```python
from build123d import *

# Parameters (mm, degrees)
F0_W     = 25.4
F0_H     = 25.4
F1_DEPTH = 44.45
F2_R     = 4.7625
F3_DEPTH = 25.401
F4_R     = 1.5875
F5_DEPTH = 12.7
F6_R     = 3.175
F7_DEPTH = 12.7


with BuildPart() as f1:
    # F0 (on Top) → F1 (new body)
    with BuildSketch(Plane.XY):
        Rectangle(F0_W, F0_H)
    extrude(amount=F1_DEPTH)

    # F2 (on face) → F3 (cut, through all)
    with BuildSketch(Plane.XZ.offset(12.7)):
        with Locations((0, 22.225)):
            Circle(F2_R)
    extrude(amount=-F3_DEPTH, mode=Mode.SUBTRACT)

    # F4 (on face) → F5 (cut)
    with BuildSketch(Plane.YZ.offset(12.7)):
        with Locations((0, 22.225)):
            Circle(F4_R)
    extrude(amount=-F5_DEPTH, mode=Mode.SUBTRACT)

    # F6 (on face) → F7 (cut)
    with BuildSketch(Plane(origin=(-12.7, 0, 0), x_dir=(0, -1, 0), z_dir=(-1, 0, 0))):
        with Locations((0, 33.3375)):
            Circle(F6_R)
        with Locations((0, 11.1125)):
            Circle(F6_R)
    extrude(amount=-F7_DEPTH, mode=Mode.SUBTRACT)


solid = f1.part
```
Geometry: final body of the model. Coordinates: model frame, mm. A direction names the side the tool comes from. Coordinates: 2 decimals unless noted, no trailing zeros. Order: outer loops, then holes, each group sorted by start corner. A loop starts at its lowest first (then second) coordinate and runs counter-clockwise, first axis right, second up. Notation, with made-up numbers: (-12, 22) - (37, 22) arc R13 ccw to (37, 47) - close; hole circle Ø5 at (4.25, 75.25). An arc over 180 degrees is marked (long way). Write each question's results on one line, items separated by ' | '.
1) Line query: line 1 (Z direction, x = 0, y = 5.75); line 2 (Z direction, x = 10.25, y = 0); line 3 (X direction, y = 6.5, z = 18). Output: solid intervals per line, ascending. Write a range as from..to.
Results list:
line 1: 0..17.46, 26.99..44.45 | line 2: 0..20.64, 23.81..44.45 | line 3: -12.7..-2.2, 2.2..12.7
2) Section B-B, the plane x = -3.25. State how many separate pieces and enclosed holes the cut face has, plus the area to 3 significant figures.
Results list:
separate pieces: 2 | enclosed holes: 2 | area: 889 mm^2
3) Section A-A, the plane x = 3.25. Return loops of the section in (y, z).
Results list:
outline: (-12.7, 0) - (12.7, 0) - (12.7, 18.74) - (-12.7, 18.74) - close; (-12.7, 25.71) - (12.7, 25.71) - (12.7, 44.45) - (-12.7, 44.45) - close
4) Pin query (flat end, axial travel): pin 1 (1.9 mm diameter, centred on y = 1, z = 10.5, fed in from -X). Return the tip coordinate at first contact, or that it passes through.
Results list:
pin 1: x = 0
5) Pull-direction query (Z, two-part tool) for faces 4 (the flat face through (0, 0, 44.45)), 5 (the flat face through (0, 0, 11)), 6 (the flat face through (-12.7, 0, 22)); classes: pulls with the +Z half, pulls with the -Z half, needs draft (parallel to the pull), parting line crosses it, or undercut.
Results list:
face 4: pulls with the +Z half | face 5: undercut | face 6: needs draft
6) Set-up query: faces 1 (the cylindrical face through (-6.439, 0.688, 8.013)), 2 (the cylindrical face through (8.652, 0.853, 23.564)), 3 (the cylindrical face through (-4.76, -0.18, 22.43)). Return all of +Z, -Z, +X, -X, +Y, -Y with unobstructed straight access to the full face (end or side cutting, diameter ignored); none if empty.
Results list:
face 1: -X | face 2: +X | face 3: +Y, -Y
